Input: part model. Units: mm. Frame: model coordinates. Give positions to 0.01 mm unless a question says otherwise; leave off trailing zeros. Write each loop counter-clockwise with the first axis right and the second up, starting at its lowest first coordinate (ties: lowest second). Pieces come first, ordered by that corner, then holes.
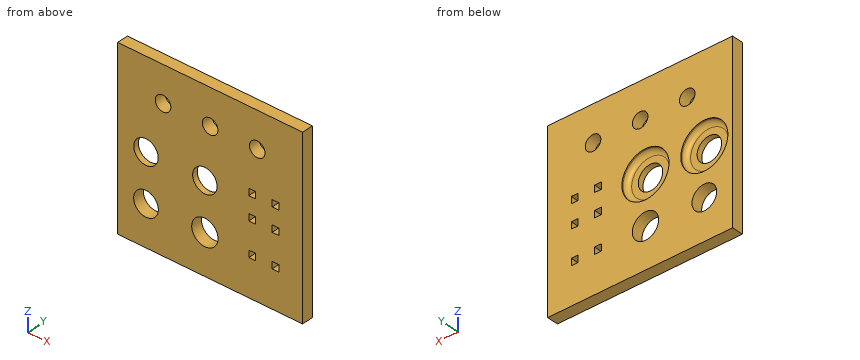
```python
from build123d import *

# Parameters (mm, degrees)
F0_W     = 78.5
F0_H     = 75
F1_DEPTH = 4.8
F2_R     = 5.2
F2_R_2   = 5.25
F2_R_3   = 5.59
F2_R_4   = 3.3
F2_W     = 2.9
F2_H     = 2.9
F3_DEPTH = 4.801
F4_R     = 10
F5_DEPTH = 2.5
F6_R     = 2


with BuildPart() as f1:
    # F0 (on Front) → F1 (new body)
    with BuildSketch(Plane.XZ):
        Rectangle(F0_W, F0_H)
    extrude(amount=F1_DEPTH)

    # F2 (on face) → F3 (cut, through all)
    with BuildSketch(Plane.XZ.offset(4.8)):
        with Locations((-27.25, 0)):
            Circle(F2_R)
        with Locations((-27.25, -20.25)):
            Circle(F2_R_2)
        with Locations((-2.25, -20.25)):
            Circle(F2_R_3)
        with Locations((-2.25, 0)):
            Circle(F2_R)
        with Locations((0, 22.2)):
            Circle(F2_R_4)
        with Locations((-20, 22.2)):
            Circle(F2_R_4)
        with Locations((20, 22.2)):
            Circle(F2_R_4)
        with Locations((17.9, 3.948761)):
            Rectangle(F2_W, F2_H)
        with Locations((27.8, 3.948761)):
            Rectangle(F2_W, F2_H)
        with Locations((17.9, -5.951239)):
            Rectangle(F2_W, F2_H)
        with Locations((27.8, -5.951239)):
            Rectangle(F2_W, F2_H)
        with Locations((17.9, -20.25)):
            Rectangle(F2_W, F2_H)
        with Locations((27.8, -20.25)):
            Rectangle(F2_W, F2_H)
    extrude(amount=-F3_DEPTH, mode=Mode.SUBTRACT)

    # F4 (on face) → F5 (cut)
    with BuildSketch(Plane(origin=(0, 0, 0), x_dir=(-1, 0, 0), z_dir=(0, 1, 0))):
        with Locations((2.25, 0)):
            Circle(F4_R)
        with Locations((27.25, 0)):
            Circle(F4_R)
    extrude(amount=-F5_DEPTH, mode=Mode.SUBTRACT)

    # F6
    f6_edges = [f1.edges().sort_by_distance(p)[0] for p in [
        (7.75, -2.5, 0),
        (-17.25, -2.5, 0),
    ]]
    fillet(f6_edges, radius=F6_R)


solid = f1.part
```
Q1. Section B-B, the plane z = 22.2. Return the cut outline in (x, y).
Q2. Section C-C, the plane x = -27.25. Return the cut outline in (y, z), then the cut area to 3 significant figures.
Q3. Section D-D, the plane x = 20.5. Return the cut outline in (y, z).
Q4. Section A-A, the plane z = 0. Return the cut outline in (x, y), then the cut area to 3 significant figures.
Q5. Pin query (flat end, axial travel): pin 1 (5.5 mm diameter, centred on x = 0, z = 22.2, fed in from +Y); pin 2 (8 mm diameter, centred on x = -6, z = -0.5, fed in from +Y). Return the tip coordinate at first contact, or that it passes through.
Q6. Material intervals for line 1 along Z through (x, y) = (-27.25, -3.4); line 2 along Z through (x, y) = (-2.25, -3.55); line 3 along X through (y, z) = (-0.15, -25), sorted ascending.
Solutions:
1. outline: (-39.25, -4.8) - (-23.3, -4.8) - (-23.3, 0) - (-39.25, 0) - close; (-16.7, -4.8) - (-3.3, -4.8) - (-3.3, 0) - (-16.7, 0) - close; (3.3, -4.8) - (16.7, -4.8) - (16.7, 0) - (3.3, 0) - close; (23.3, -4.8) - (39.25, -4.8) - (39.25, 0) - (23.3, 0) - close
2. outline: (-4.8, -37.5) - (0, -37.5) - (0, -25.5) - (-4.8, -25.5) - close; (-4.8, -15) - (0, -15) - (0, -10) - (-0.5, -10) arc R2 cw to (-2.5, -8) - (-2.5, -5.2) - (-4.8, -5.2) - close; (-4.8, 5.2) - (-2.5, 5.2) - (-2.5, 8) arc R2 cw to (-0.5, 10) - (0, 10) - (0, 37.5) - (-4.8, 37.5) - close
2. area: 237 mm2
3. outline: (-4.8, -37.5) - (0, -37.5) - (0, 18.94) - (-4.8, 18.94) - close; (-4.8, 25.46) - (0, 25.46) - (0, 37.5) - (-4.8, 37.5) - close
4. outline: (-39.25, -4.8) - (-32.45, -4.8) - (-32.45, -2.5) - (-35.25, -2.5) arc R2 cw to (-37.25, -0.5) - (-37.25, 0) - (-39.25, 0) - close; (-22.05, -4.8) - (-7.45, -4.8) - (-7.45, -2.5) - (-10.25, -2.5) arc R2 cw to (-12.25, -0.5) - (-12.25, 0) - (-17.25, 0) - (-17.25, -0.5) arc R2 cw to (-19.25, -2.5) - (-22.05, -2.5) - close; (2.95, -4.8) - (39.25, -4.8) - (39.25, 0) - (7.75, 0) - (7.75, -0.5) arc R2 cw to (5.75, -2.5) - (2.95, -2.5) - close
4. area: 232 mm2
5. pin 1: passes through
5. pin 2: stops at y = -2.5
6. line 1: z = -37.5 to -25.5, -15 to -5.2, 5.2 to 37.5
6. line 2: z = -37.5 to -25.84, -14.66 to -5.2, 5.2 to 19.79, 24.61 to 37.5
6. line 3: x = -39.25 to -29.49, -25.01 to -5.2, 0.7 to 39.25
